Work out the finished part from the listing and answer in its coordinate system (mm). A direction names the side the tool comes from. Round coordinates to 2 decimals unless told otherwise and drop trailing zeros. Order: outer loops, then holes, each group sorted by start corner. A loop starts at its lowest first (then second) coordinate and runs counter-clockwise, first axis right, second up. Notation, with made-up numbers: M -9.5,-31 L -3.5,-31 A21 ccw -3.5,-27 Z; hole C -6,65.25 d5. An arc over 180 degrees is marked long. Return JSON: item names as keys, results as strings.
from build123d import *

# Parameters (mm, degrees)
F0_R          = 3.375
F1_DEPTH      = 6
F2_W          = 8.3882776671
F2_H          = 17.9039358627
F3_DEPTH      = 4.576
F3_DEPTH_BACK = 25
F4_T1_DEPTH   = 13.2089304981
F4_T3_DEPTH   = 11.8980683562
F5_R          = 0.5
F6_T1_DEPTH   = 1.9309283779
F6_T3_DEPTH   = 2.3257264643
F6_T8_ANGLE   = 73.0382941175
F6_T10_ANGLE  = 81.5443380081
F6_T12_ANGLE  = 196.5215831172


# Not quite as in the source:
# - a fillet or chamfer that OpenCascade refuses, or shapes differently, is made with other operations: its cross-section is extruded or revolved along the edge and cut away or added


with BuildPart() as f1:
    # F0 (on Front) → F1 (new body)
    with BuildSketch(Plane.XZ):
        with BuildLine():
            Line((0, 15), (-4.575, 0))
            ThreePointArc((-4.575, 0), (0.7061497994, -4.5201744945), (4.3570120047, 1.395375))
            Line((4.3570120047, 1.395375), (0, 15))
        make_face()
        Circle(F0_R, mode=Mode.SUBTRACT)
    extrude(amount=F1_DEPTH)

    # F2 (on Right) → F3 (cut, two sides)
    with BuildSketch(Plane.YZ) as f3_sk:
        with Locations((-4.7752561222, 12.6100402558)):
            Rectangle(F2_W, F2_H)
    extrude(amount=-F3_DEPTH, mode=Mode.SUBTRACT)
    extrude(f3_sk.sketch, amount=F3_DEPTH_BACK, mode=Mode.SUBTRACT)

    # F4: fillet of radius 3.5 on 2 edges, made by hand

    # F4_s2 → F4_t1 (cut)
    with BuildSketch(Plane.XZ.offset(0.5811172887)):
        with BuildLine():
            ThreePointArc((4.5252695152, 0.6727264041), (3.3489995726, 2.8086655863), (1.0633146948, 3.6580723245))
            Line((1.0633146948, 3.6580723245), (1.0633146948, 4.0080723245))
            Line((1.0633146948, 4.0080723245), (3.6323614241, 4.0080723245))
            Line((3.6323614241, 4.0080723245), (3.9656847468, 3.7648223245))
            ThreePointArc((3.9656847468, 3.7648223245), (4.6903353275, 1.502125), (4.8714649972, 0.7241918121))
            Line((4.8714649972, 0.7241918121), (4.5252695152, 0.6727264041))
        make_face()
    extrude(amount=F4_T1_DEPTH, mode=Mode.SUBTRACT)

    # F4_s4 → F4_t3 (cut)
    with BuildSketch(Plane.XZ.offset(0.5811172887)):
        with BuildLine():
            ThreePointArc((-4.2153635131, 1.1791360226), (-2.9504335333, 2.9708754587), (-0.8676136831, 3.6580723245))
            Line((-0.8676136831, 3.6580723245), (-3.459287941, 3.6580723245))
            Line((-3.459287941, 3.6580723245), (-4.2153635131, 1.1791360226))
        make_face()
    extrude(amount=F4_T3_DEPTH, mode=Mode.SUBTRACT)

    # F5
    f5_edges = [f1.edges().sort_by_distance(p)[0] for p in [
        (0, -0.290559, 15),
    ]]
    fillet(f5_edges, radius=F5_R)

    # F6: chamfer of 0.25 on 6 edges, made by hand

    # F6_s2 → F6_t1 (cut)
    with BuildSketch(Plane.YZ.offset(-0.8676136831)):
        Polygon((-6, 3.4080723245), (-5.75, 3.6580723245), (-6, 3.6580723245), align=None)
    extrude(amount=F6_T1_DEPTH, mode=Mode.SUBTRACT)

    # F6_s4 → F6_t3 (cut)
    with BuildSketch(Plane(origin=(-0.0297318944, 0, -0.0974816211), x_dir=(0, 1, 0), z_dir=(-0.2917324852, 0, -0.9564999514))):
        Polygon((-5.75, -4.3759872778), (-6, -4.1259872778), (-6, -4.3759872778), align=None)
    extrude(amount=F6_T3_DEPTH, mode=Mode.SUBTRACT)

    # F6_s5 → F6_t6 (revolve, cut)
    with BuildSketch(Plane.XY):
        Polygon((3.375, -5.75), (3.625, -6), (3.375, -6), align=None)
    revolve(axis=Axis((0, -6, 0), (0, -1, 0)), mode=Mode.SUBTRACT)

    # F6_s7 → F6_t8 (revolve, cut)
    with BuildSketch(Plane(origin=(-0.0297318944, 0, -0.0974816209), x_dir=(0, 1, 0), z_dir=(-0.2917324851, 0, -0.9564999514))):
        Polygon((-6, -4.1259872778), (-5.75, -4.3759872778), (-6, -4.3759872778), align=None)
    revolve(axis=Axis((-0.8676136832, -6, 0.1580723246), (0, 1, 0)), revolution_arc=F6_T8_ANGLE, mode=Mode.SUBTRACT)

    # F6_s9 → F6_t10 (revolve, cut)
    with BuildSketch(Plane.YZ.offset(1.0633146948)):
        Polygon((-5.75, 3.6580723245), (-6, 3.4080723245), (-6, 3.6580723245), align=None)
    revolve(axis=Axis((1.0633146948, -6, 0.1580723245), (0, 1, 0)), revolution_arc=F6_T10_ANGLE, mode=Mode.SUBTRACT)

    # F6_s11 → F6_t12 (revolve, cut)
    with BuildSketch(Plane(origin=(0, 0, 0), x_dir=(0, 1, 0), z_dir=(0.1403123523, 0, 0.990107289))):
        Polygon((-5.75, 4.575), (-6, 4.325), (-6, 4.575), align=None)
    revolve(axis=Axis((0, -6, 0), (0, -1, 0)), revolution_arc=F6_T12_ANGLE, mode=Mode.SUBTRACT)


solid = f1.part
Item 1: Find section C-C (z = 10.75). Determine the outline of the cut face in (x, y).
Output:
{"outline": "M -1.3,-0.58 L 1.36,-0.58 L 1.36,0 L -1.3,0 Z"}
Item 2: Consider line 1 along Z through (x, y) = (0, -1.2) (3 decimals); line 2 along Y through (x, z) = (0.25, 8); line 3 along X through (y, z) = (-1.5, -0.75). Determine where each line is inside the solid, lowest interval first. Write a range as [from, to].
Output:
{"line 1": "z = [-4.575, -3.375], [3.375, 3.658]", "line 2": "y = [-0.58, 0]", "line 3": "x = [-4.51, -3.29], [3.29, 4.51]"}
Item 3: Find section A-A (y = -3.5). Determine the outline of the cut face in (x, z) (3 decimals), plus the area to 3 significant figures.
Output:
{"outline": "M -4.575,0 A4.575 ccw long 4.525,0.673 A3.5 ccw 1.063,3.658 L -0.868,3.658 A3.5 ccw -4.215,1.179 Z; hole C 0,0 d6.75", "area": "24.6 mm^2"}
Item 4: Find section D-D (z = 8.75). Determine the outline of the cut face in (x, y).
Output:
{"outline": "M -1.91,-0.58 L 2,-0.58 L 2,0 L -1.91,0 Z"}
Item 5: Each of these flat-tipped pins is pushed along its axis until it touches: pin 1 (1.5 mm diameter, centred on y = -4, z = 2.5, fed in from +X); pin 2 (2 mm diameter, centred on x = -3.5, y = -2, fed in from +Z); pin 3 (1.5 mm diameter, centred on x = 0, y = -3.5, fed in from +Z). Where does it stop, or does it pass through?
Output:
{"pin 1": "stops at x = 4.18", "pin 2": "stops at z = 3.25", "pin 3": "stops at z = 3.66"}
Item 6: The mould has two halves that part along Z. Classify faces 4 (the cylindrical face through (3.375, -3.129, 2.786)), 5 (the flat face through (0, 0, 5)), 6 (the cylindrical face through (-0.7, -2.8, -3.3)): pulls with the +Z half, pulls with the -Z half, needs draft (parallel to the pull), parting line crosses it, or undercut.
Output:
{"face 4": "pulls with the +Z half", "face 5": "needs draft", "face 6": "undercut"}
Item 7: Find section B-B (x = 0). Determine the outline of the cut face in (y, z) (3 decimals), plus the area to 3 significant figures.
Output:
{"outline": "M -6,-4.325 L -5.75,-4.575 L 0,-4.575 L 0,-3.375 L -5.75,-3.375 L -6,-3.625 Z; M -5.892,3.517 L -5.75,3.375 L 0,3.375 L 0,13.824 L -0.581,13.824 L -0.581,3.658 L -5.75,3.658 Z", "area": "14.7 mm^2"}
Item 8: Which of the six approach directions +Z, -Z, +X, -X, +Y, -Y give full straight-line access (tool end or side, diameter ignored) to faces 1 (the flat face through (2.45, -0.29, 7.35)), 2 (the flat face through (0, -3, 3.658)), 3 (the cylindrical face through (-2.98, -3.13, 2.95))?
Output:
{"face 1": "+Z, +X, +Y, -Y", "face 2": "+Z, +X, -X, -Y", "face 3": "+Z, -X, -Y"}
